Study the drawing (mm; zero at the part's minimum x, y, z) and answer. A direction names the side the tool comes from. Coordinates: 2 decimals unless noted, no trailing zeros. Order: outer loops, then holes, each group sorted by start corner. A loop starts at its lowest first (then second) coordinate and runs counter-clockwise, first axis right, second up. Notation, with made-up numbers: M -2.5,3.5 L 35.5,3.5 A4 cw 35.5,8.5 Z; hole C -35.5,33 d7. An arc over 180 degrees is marked long. Use a Markdown table: item, result. Add a question column.
1) Find the intervals of material crossed by probe 1 along Y at (x, z) = (0.95, 10.7); probe 2 along X at (y, z) = (3.15, 12.5), in increasing order. Write a range as [from, to].
2) The mould has two halves that part along Y. Classify the marked faces 3, 4, 5 and 6: released by +Y, released by -Y, zero draft, split by the parting line, or undercut.
3) Find section B-B on x = 7.5. Write down the section's boundary in (y, z) (1 decimal).
4) Find section C-C on z = 10.7. Write down the section's boundary in (x, y).
5) Find section A-A on y = 2.8. Write down the section's boundary in (x, z) (1 decimal).
6) Find section D-D on y = 2.15. Write down the section's boundary in (x, z) (1 decimal).
7) For the marked faces 1 and 2, determine the directions among +Z, -Z, +X, -X, +Y, -Y from which every point of the face is accessible in a straight line to the end or side of a thin tool.
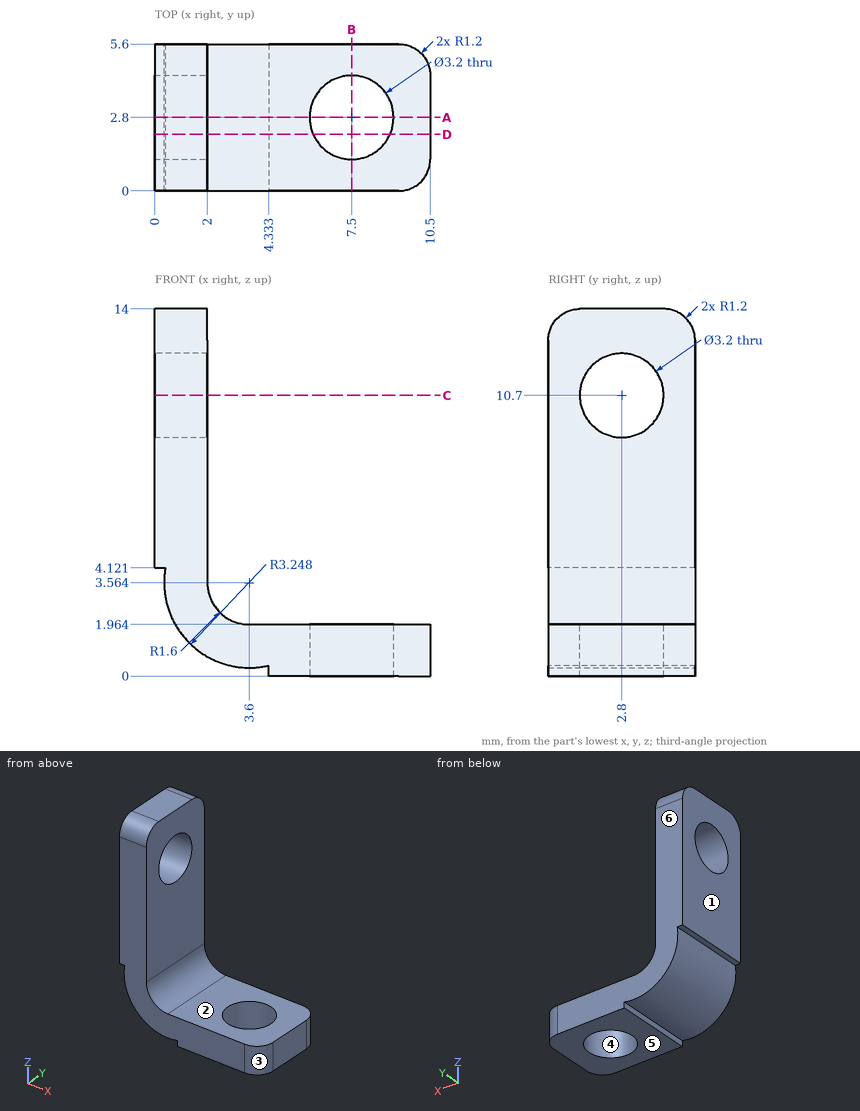
Check result:
| question | item | result |
|---|---|---|
| 1 | probe 1 | y = [0, 1.2], [4.4, 5.6] |
| 1 | probe 2 | x = [0, 2] |
| 2 | face 3 | released by -Y |
| 2 | face 4 | undercut |
| 2 | face 5 | zero draft |
| 2 | face 6 | released by +Y |
| 3 | outline | M 0,0 L 1.2,0 L 1.2,2 L 0,2 Z; M 4.4,0 L 5.6,0 L 5.6,2 L 4.4,2 Z |
| 4 | outline | M 0,0 L 2,0 L 2,1.2 L 0,1.2 Z; M 0,4.4 L 2,4.4 L 2,5.6 L 0,5.6 Z |
| 5 | outline | M 0,4.1 L 0.4,4.1 A3.2 ccw 4.3,0.4 L 4.3,0 L 5.9,0 L 5.9,2 L 3.6,2 A1.6 cw 2,3.6 L 2,9.1 L 0,9.1 Z; M 0,12.3 L 2,12.3 L 2,14 L 0,14 Z; M 9.1,0 L 10.5,0 L 10.5,2 L 9.1,2 Z |
| 6 | outline | M 0,4.1 L 0.4,4.1 A3.2 ccw 4.3,0.4 L 4.3,0 L 6,0 L 6,2 L 3.6,2 A1.6 cw 2,3.6 L 2,9.2 L 0,9.2 Z; M 0,12.2 L 2,12.2 L 2,14 L 0,14 Z; M 9,0 L 10.5,0 L 10.5,2 L 9,2 Z |
| 7 | face 1 | +Z, -Z, -X, +Y, -Y |
| 7 | face 2 | +Z, +X, +Y, -Y |
